Model file for the job. Use its own axes, mm. Give positions to 0.01 mm unless a question says otherwise; leave off trailing zeros. Write each loop counter-clockwise with the first axis right and the second up, starting at its lowest first coordinate (ties: lowest second). Pieces come first, ordered by that corner, then holes. Notation, with made-up numbers: (26.25, -25) - (48.25, -25) arc R36 cw to (48.25, 11) - close; hole circle Ø7 at (87.5, 25). An arc over 180 degrees is marked (long way). Use a Markdown table: item, result. Add a question column.
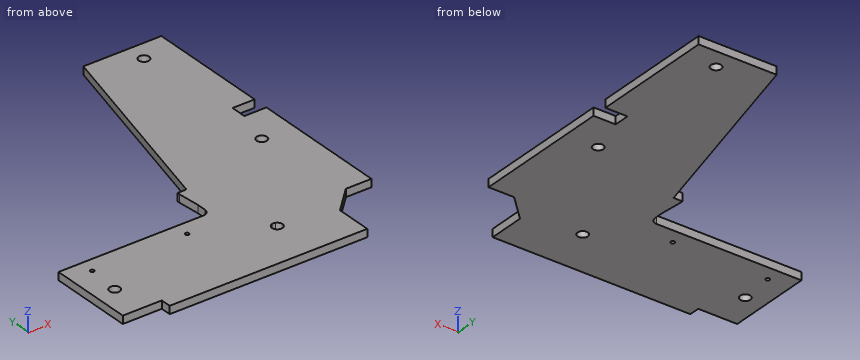
```python
from build123d import *

# Parameters (mm, degrees)
BOSS_EXTRUDE2_DEPTH     = 6
SKETCH2_R               = 4
SKETCH2_W               = 30
SKETCH2_H               = 8.3
CUT_EXTRUDE1_DEPTH      = 341.487943986
CROQUIS1_W              = 103.610606389
CROQUIS1_H              = 1.56
SALIENTE_EXTRUIR2_DEPTH = 6
SALIENTE_EXTRUIR3_DEPTH = 6
SALIENTE_EXTRUIR4_START = -6
SALIENTE_EXTRUIR4_DEPTH = 6
SALIENTE_EXTRUIR5_DEPTH = 6
SALIENTE_EXTRUIR6_DEPTH = 6
CROQUIS7_W              = 103.610606389
CROQUIS7_H              = 0.56
SALIENTE_EXTRUIR7_DEPTH = 6
SALIENTE_EXTRUIR8_DEPTH = 6
SKETCH3_R               = 1.5
CUT_EXTRUDE2_DEPTH      = 341.487943986
CUT_EXTRUDE3_DEPTH      = 341.487943986
CROQUIS9_W              = 152
CROQUIS9_H              = 0.3
CORTAR_EXTRUIR1_DEPTH   = 10
CORTAR_EXTRUIR2_DEPTH   = 6
CROQUIS12_R             = 4
CORTAR_EXTRUIR3_DEPTH   = 6
SALIENTE_EXTRUIR9_DEPTH = 6
CROQUIS14_W             = 17
CROQUIS14_H             = 12
CORTAR_EXTRUIR4_DEPTH   = 10


with BuildPart() as part:
    # Sketch1 → Boss-Extrude2 (new body)
    with BuildSketch(Plane.XY):
        with BuildLine():
            Line((0, 0), (-220, 0))
            Line((-220, 0), (-220, 71.45))
            Line((-220, 71.45), (-116.389393611, 71.45))
            ThreePointArc((-116.389393611, 71.45), (-107.149394721, 74.662079518), (-101.894274329, 82.913063942))
            Line((-101.894274329, 82.913063942), (-60, 259.8))
            Line((-60, 259.8), (0, 259.8))
            Line((0, 259.8), (0, 0))
        make_face()
    extrude(amount=BOSS_EXTRUDE2_DEPTH)

    # Sketch2 → Cut-Extrude1 (cut, through all)
    with BuildSketch(Plane.XY.offset(6)):
        with Locations((-205, 36.3)):
            Circle(SKETCH2_R)
        with Locations((-24.8, 244.8)):
            Circle(SKETCH2_R)
        with Locations((-24.8, 125)):
            Circle(SKETCH2_R)
        with Locations((-80, 43.8)):
            Circle(SKETCH2_R)
        with Locations((-205, 4.15)):
            Rectangle(SKETCH2_W, SKETCH2_H)
        Polygon((-38, 0), (-38, 19), (-10.7, 46.3), (0, 46.3), (0, 0), align=None)
    extrude(amount=-CUT_EXTRUDE1_DEPTH, mode=Mode.SUBTRACT)

    # Croquis1 → Saliente-Extruir2 (add)
    with BuildSketch(Plane.XY.offset(6)):
        with Locations((-168.194696806, 72.23)):
            Rectangle(CROQUIS1_W, CROQUIS1_H)
    extrude(amount=-SALIENTE_EXTRUIR2_DEPTH)

    # Croquis3 → Saliente-Extruir3 (add)
    with BuildSketch(Plane.XY.offset(6)):
        Polygon((-101.894274329, 82.913063942), (-103.412279578, 83.272591501), (-60, 259.8), align=None)
    extrude(amount=-SALIENTE_EXTRUIR3_DEPTH)

    # Croquis4 → Saliente-Extruir4 (add)
    with BuildSketch(Plane.XY.offset(6).offset(SALIENTE_EXTRUIR4_START)):
        with BuildLine():
            Line((-103.412279578, 83.272591501), (-101.894274329, 82.913063942))
            ThreePointArc((-101.894274329, 82.913063942), (-107.149394721, 74.662079518), (-116.389393611, 71.45))
            Line((-116.389393611, 71.45), (-116.389393611, 73.01))
            ThreePointArc((-116.389393611, 73.01), (-108.117056079, 75.88569363), (-103.412279578, 83.272591501))
        make_face()
    extrude(amount=SALIENTE_EXTRUIR4_DEPTH)

    # Croquis5 → Saliente-Extruir5 (add)
    with BuildSketch(Plane.XY.offset(6)):
        Polygon((-105, 102.74), (-55, 102.74), (-103.412279578, 83.272591501), align=None)
    extrude(amount=-SALIENTE_EXTRUIR5_DEPTH)

    # Croquis6 → Saliente-Extruir6 (add)
    with BuildSketch(Plane.XY.offset(6)):
        Polygon((-98.157526679, 104.64), (-105.154959958, 104.64), (-105, 102.74), (-98.624781775, 102.74), align=None)
    extrude(amount=-SALIENTE_EXTRUIR6_DEPTH)

    # Croquis7 → Saliente-Extruir7 (add)
    with BuildSketch(Plane.XY.offset(6)):
        with Locations((-168.194696806, 73.29)):
            Rectangle(CROQUIS7_W, CROQUIS7_H)
    extrude(amount=-SALIENTE_EXTRUIR7_DEPTH)

    # Croquis8 → Saliente-Extruir8 (add)
    with BuildSketch(Plane.XY.offset(6)):
        with BuildLine():
            Line((-116.389393611, 73.57), (-117.98880457, 71.652693326))
            Line((-117.98880457, 71.652693326), (-105.380568296, 73.057716723))
            Line((-105.380568296, 73.057716723), (-100.684832206, 83.373546401))
            Line((-100.684832206, 83.373546401), (-103.622774874, 85.853523162))
            ThreePointArc((-103.622774874, 85.853523162), (-107.531184208, 77.13952683), (-116.389393611, 73.57))
        make_face()
    extrude(amount=-SALIENTE_EXTRUIR8_DEPTH)

    # Sketch3 → Cut-Extrude2 (cut, through all)
    with BuildSketch(Plane.XY.offset(6)):
        with Locations((-202.75, 62.07)):
            Circle(SKETCH3_R)
        with Locations((-129.75, 62.07)):
            Circle(SKETCH3_R)
    extrude(amount=-CUT_EXTRUDE2_DEPTH, mode=Mode.SUBTRACT)

    # Sketch4 → Cut-Extrude3 (cut, through all)
    with BuildSketch(Plane.XY.offset(6)):
        with BuildLine():
            Line((-103.622774874, 85.853523162), (-103.622774874, 78.57))
            ThreePointArc((-103.622774874, 78.57), (-105.087240968, 75.034466094), (-108.622774874, 73.57))
            Line((-108.622774874, 73.57), (-116.389393611, 73.57))
            ThreePointArc((-116.389393611, 73.57), (-107.531184208, 77.13952683), (-103.622774874, 85.853523162))
        make_face()
    extrude(amount=-CUT_EXTRUDE3_DEPTH, mode=Mode.SUBTRACT)

    # Croquis9 → Cortar-Extruir1 (cut)
    with BuildSketch(Plane.XY.offset(6)):
        with Locations((-114, 0.15)):
            Rectangle(CROQUIS9_W, CROQUIS9_H)
    extrude(amount=-CORTAR_EXTRUIR1_DEPTH, mode=Mode.SUBTRACT)

    # Croquis11 → Cortar-Extruir2 (cut)
    with BuildSketch(Plane.XY.offset(6)):
        Polygon((-10.7, 46.3), (-19.7, 46.3), (-38, 28), (-38, 19), align=None)
    extrude(amount=-CORTAR_EXTRUIR2_DEPTH, mode=Mode.SUBTRACT)

    # Croquis12 → Cortar-Extruir3 (cut)
    with BuildSketch(Plane.XY.offset(6)):
        with Locations((-80, 36.3)):
            Circle(CROQUIS12_R)
    extrude(amount=-CORTAR_EXTRUIR3_DEPTH, mode=Mode.SUBTRACT)

    # Croquis13 → Saliente-Extruir9 (add)
    with BuildSketch(Plane.XY.offset(6)):
        with BuildLine():
            ThreePointArc((-78.608058909, 40.05), (-76.716117819, 41.516117819), (-76, 43.8))
            ThreePointArc((-76, 43.8), (-82.283882181, 47.083882181), (-81.391941091, 40.05))
            ThreePointArc((-81.391941091, 40.05), (-80, 40.3), (-78.608058909, 40.05))
        make_face()
    extrude(amount=-SALIENTE_EXTRUIR9_DEPTH)

    # Croquis14 → Cortar-Extruir4 (cut)
    with BuildSketch(Plane.XY.offset(6)):
        with Locations((-8.5, 159.05)):
            Rectangle(CROQUIS14_W, CROQUIS14_H)
    extrude(amount=-CORTAR_EXTRUIR4_DEPTH, mode=Mode.SUBTRACT)


solid = part.part
```
(1) Band-saw the part on A-A (x = -24.8). Write the cut outline in (y, z).
(2) Flat gauge pins, fed straight in: pin 1 (2 mm diameter, centred on x = -144, z = 2, fed in from +Y); pin 2 (6.5 mm diameter, centred on x = -24.8, y = 244.8, fed in from +Z); pin 3 (3 mm diameter, centred on x = -103, z = 3.5, fed in from +Y). Where does each tip first touch, or does it go through?
(3) Band-saw the part on C-C (y = 125). Write the cut outline in (x, z), then the cut area to 3 significant figures.
(4) Probe probe 1 along Y at (x, z) = (-205, 3.25); probe 2 along Y at (x, z) = (-27.5, 2.1); probe 3 along Y at (x, z) = (-164, 1.9). List the from-to ranges inside material, lowest first. Write a range as [from, to].
(5) Band-saw the part on D-D (y = 17.5). Write the cut outline in (x, z), then the cut area to 3 significant figures.
(6) Band-saw the part on B-B (z = 1.9). Write the cut outline in (x, y), then the cut area to 3 significant figures.
Model answer:
| question | item | result |
|---|---|---|
| 1 | outline | (41.2, 0) - (121, 0) - (121, 6) - (41.2, 6) - close; (129, 0) - (240.8, 0) - (240.8, 6) - (129, 6) - close; (248.8, 0) - (259.8, 0) - (259.8, 6) - (248.8, 6) - close |
| 2 | pin 1 | stops at y = 73.57 |
| 2 | pin 2 | passes through |
| 2 | pin 3 | stops at y = 104.64 |
| 3 | outline | (-93.15, 0) - (-28.8, 0) - (-28.8, 6) - (-93.15, 6) - close; (-20.8, 0) - (0, 0) - (0, 6) - (-20.8, 6) - close |
| 3 | area | 511 mm^2 |
| 4 | probe 1 | y = [8.3, 32.3], [40.3, 73.57] |
| 4 | probe 2 | y = [38.5, 122.05], [127.95, 241.85], [247.75, 259.8] |
| 4 | probe 3 | y = [0.3, 73.57] |
| 5 | outline | (-220, 0) - (-38, 0) - (-38, 6) - (-220, 6) - close |
| 5 | area | 1,090 mm^2 |
| 6 | outline | (-220, 8.3) - (-190, 8.3) - (-190, 0.3) - (-38, 0.3) - (-38, 28) - (-19.7, 46.3) - (0, 46.3) - (0, 153.05) - (-17, 153.05) - (-17, 165.05) - (0, 165.05) - (0, 259.8) - (-60, 259.8) - (-98.16, 104.64) - (-105.15, 104.64) - (-103.62, 85.85) - (-103.62, 78.57) arc R5 cw to (-108.62, 73.57) - (-220, 73.57) - close; hole circle Ø8 at (-205, 36.3); hole circle Ø3 at (-202.75, 62.07); hole circle Ø3 at (-129.75, 62.07); hole circle Ø8 at (-80, 36.3); hole circle Ø8 at (-24.8, 125); hole circle Ø8 at (-24.8, 244.8) |
| 6 | area | 29,400 mm^2 |
